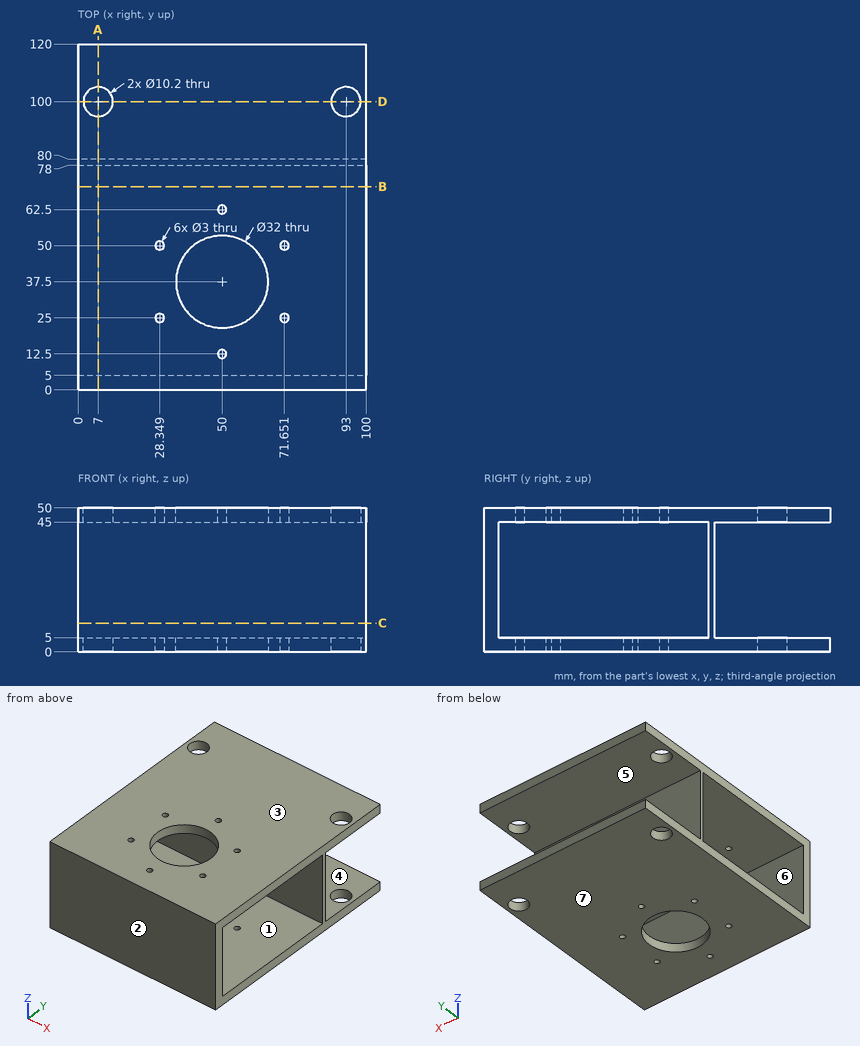
Geometry check sheet. Reference: drawing and pictorial views, mm from the part's lowest x, y, z. A direction names the side the tool comes from. Coordinates: 2 decimals unless noted, no trailing zeros. Order: outer loops, then holes, each group sorted by start corner. A loop starts at its lowest first (then second) coordinate and runs counter-clockwise, first axis right, second up.
Item 1: Section check A-A (x = 7). Enter the section's corners in (y, z).
Item 2: Section check C-C (z = 10). Enter the section's corners in (x, y).
Item 3: Tool access check on the marked faces 5, 6 and 7. Record the directions out of +Z, -Z, +X, -X, +Y, -Y that give a thin tool (end or side, any length) a straight path to the whole face; none if there is none.
Item 4: Section check D-D (y = 100). Enter the section's corners in (x, z), plus the area to 3 significant figures.
Item 5: Section check B-B (y = 70.5). Enter the section's corners in (x, z).
Item 6: Scan lines: line 1 along Y through (x, z) = (89.5, 31.5); line 2 along Z through (x, y) = (68, 94); line 3 along Y through (x, z) = (7, 46.7). Record each from-to range of solid material in increasing order.
Item 7: Depth check by flat-ended pin: pin 1 (4 mm diameter, centred on x = 71.65, y = 25, fed in from +Z); pin 2 (1.8 mm diameter, centred on x = 71.65, y = 25, fed in from +Z); pin 3 (12 mm diameter, centred on x = 61.5, z = 24.5, fed in from +Y). Enter the tip coordinate at first touch or a pass-through.
Item 8: Mould release check, pull along Z, two halves, no side actions. Record for the marked faces 1, 2, 3 and 4: released by +Z, released by -Z, zero draft, split by the parting line, or undercut.
Check sheet entries:
1. outline: (0, 0) - (94.9, 0) - (94.9, 5) - (80, 5) - (80, 45) - (94.9, 45) - (94.9, 50) - (0, 50) - close; (105.1, 0) - (120, 0) - (120, 5) - (105.1, 5) - close; (105.1, 45) - (120, 45) - (120, 50) - (105.1, 50) - close; hole (5, 5) - (78, 5) - (78, 45) - (5, 45) - close
2. outline: (0, 0) - (100, 0) - (100, 5) - (0, 5) - close; (0, 78) - (100, 78) - (100, 80) - (0, 80) - close
3. face 5: +X, -X, +Y
3. face 6: +X, -X
3. face 7: -Z, +X, -X, +Y, -Y
4. outline: (0, 0) - (1.9, 0) - (1.9, 5) - (0, 5) - close; (0, 45) - (1.9, 45) - (1.9, 50) - (0, 50) - close; (12.1, 0) - (87.9, 0) - (87.9, 5) - (12.1, 5) - close; (12.1, 45) - (87.9, 45) - (87.9, 50) - (12.1, 50) - close; (98.1, 0) - (100, 0) - (100, 5) - (98.1, 5) - close; (98.1, 45) - (100, 45) - (100, 50) - (98.1, 50) - close
4. area: 796 mm2
5. outline: (0, 0) - (100, 0) - (100, 5) - (0, 5) - close; (0, 45) - (100, 45) - (100, 50) - (0, 50) - close
6. line 1: y = 0 to 5, 78 to 80
6. line 2: z = 0 to 5, 45 to 50
6. line 3: y = 0 to 94.9, 105.1 to 120
7. pin 1: stops at z = 50
7. pin 2: passes through
7. pin 3: stops at y = 80
8. face 1: undercut
8. face 2: zero draft
8. face 3: released by +Z
8. face 4: undercut
